```python
from build123d import *

# Parameters (mm, degrees)
CHAMFER1_SIZE = 0.762


with BuildPart() as part:
    # Sketch1 → Base-Revolve (revolve)
    with BuildSketch(Plane.XY):
        Polygon((8.73125, 0), (8.73125, 4.7625), (6.35, 4.7625), (6.35, 2.38125), (-6.35, 2.38125), (-6.35, 4.7625), (-8.73125, 4.7625), (-8.73125, 0), align=None)
    revolve(axis=Axis((0, 0, 0), (1, 0, 0)))

    # Chamfer1
    chamfer1_edges = [part.edges().sort_by_distance(p)[0] for p in [
        (8.73125, -4.7625, 0),
        (-8.73125, -4.7625, 0),
    ]]
    chamfer(chamfer1_edges, length=CHAMFER1_SIZE)


solid = part.part
```
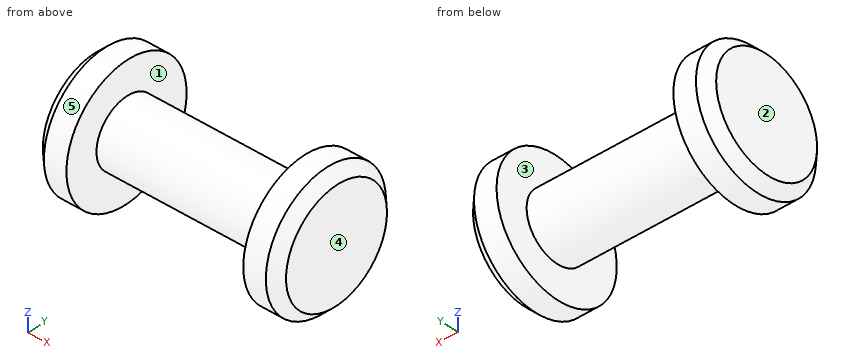
CAD build for the part. Positions are in the model's coordinates, mm. Face numbers are marked on the shaded views. A direction names the side the tool comes from. Give positions to 0.01 mm unless a question says otherwise; leave off trailing zeros. Write each loop counter-clockwise with the first axis right and the second up, starting at its lowest first coordinate (ties: lowest second). Pieces come first, ordered by that corner, then holes. Notation, with made-up numbers: (-2.5, -40) -> (11.5, -40) arc R9 cw to (11.5, -28) -> close; hole circle Ø2 at (52, -7). An arc over 180 degrees is marked (long way). Write each question's results on one line, items separated by ' | '.
1. Drop flat-ended pins along their axis: P1, Ø3, axis at x = 0, z = -0.5, coming from the -Y side; P2, Ø2, axis at x = 0, y = -1.5, coming from the +Z side. Give the stop position or say it passes through.
Geometry check:
P1: y = -2.38 | P2: z = 2.33
2. Two-plate mould, pull along X, no slides. Class the marked faces 3, 4 and 5: pulls with the +X half, pulls with the -X half, needs draft (parallel to the pull), parting line crosses it, or undercut.
Geometry check:
face 3: undercut | face 4: pulls with the +X half | face 5: needs draft
3. Cut at C-C, the plane x = 0.75. Write the cut outline in (y, z).
Geometry check:
outline: circle Ø4.76 at (0, 0)
4. Cut at A-A, the plane z = 0. Write the cut outline in (x, y), then the cut area to 3 significant figures.
Geometry check:
outline: (-8.73, -4) -> (-7.97, -4.76) -> (-6.35, -4.76) -> (-6.35, -2.38) -> (6.35, -2.38) -> (6.35, -4.76) -> (7.97, -4.76) -> (8.73, -4) -> (8.73, 4) -> (7.97, 4.76) -> (6.35, 4.76) -> (6.35, 2.38) -> (-6.35, 2.38) -> (-6.35, 4.76) -> (-7.97, 4.76) -> (-8.73, 4) -> close | area: 105 mm²
5. Which spindle directions (+Z, -Z, +X, -X, +Y, -Y) get a long thin tool onto all of the face, cutting with end or side? Do the marked faces 1 and 2. Say none if no direction does.
Geometry check:
face 1: none | face 2: +Z, -Z, -X, +Y, -Y
6. Wall check: probe 1 along X at (y, z) = (-2.25, 2); probe 2 along X at (y, z) = (-2.75, -3.75); probe 3 along Z at (x, y) = (3, 1.75). Give the ranges that are in metal, low to high. Write a range as [from, to].
Geometry check:
probe 1: [-8.73, -6.35], [6.35, 8.73] | probe 2: [-8.08, -6.35], [6.35, 8.08] | probe 3: [-1.61, 1.61]
